Autodesk Inventor part; units mm, degrees
ref_plane "Work Plane1" through (26.5484, 0, 0) normal (0, 0, -1) x (-1, 0, 0)
ref_plane "YZ Plane" through (0, 0, 0) normal (1, 0, 0) x (0, 1, 0)
ref_plane "XZ Plane" through (0, 0, 0) normal (0, 1, 0) x (-1, 0, 0)
sketch "Sketch1" plane through (0, 0, 0) normal (0, 0, 1) x (1, 0, 0)
  line L0 (-1.8762, 0) -> (9.646, 0)
  line L1 (3.3073, 6.5) -> (2.2392, 8.35)
  line L2 (3.3073, 6.5) -> (8, 6.5) construction
  line L3 (8, 6.5) -> (8, 0) construction
  arc A0 (2.2392, 8.35) -> (0, 7.75) centre (1.2, 7.75) ccw
  line L4 (3.3073, 6.5) -> (3.3073, 0)
  line L5 (0, -1.8418) -> (0, 11.0509)
  point P0 (0, 0)
  dimension "d2" = 13
  dimension "d4" = 17.9
  dimension "d5" = 1.2
  dimension "d15" = 8
  dimension "d16" = 30
revolve "Ring" add sketch "Sketch1" angle 360 about axis through (-10, 0, 0) along (1, 0, 0)
sketch "Sketch2" plane through (0, 0, 0) normal (-1, 0, 0) x (0, 0, 1)
  circle A0 centre (0, 0) radius 4.9
  line L0 (-6.5, -3.7528) -> (-6.5, 3.7528)
  line L1 (-6.5, 3.7528) -> (0, 7.5056)
  line L2 (0, 7.5056) -> (6.5, 3.7528)
  line L3 (6.5, 3.7528) -> (6.5, -3.7528)
  line L4 (6.5, -3.7528) -> (0, -7.5056)
  line L5 (0, -7.5056) -> (-6.5, -3.7528)
  circle A1 centre (0, 0) radius 7.75
  dimension "d6" = 15.0111
extrude "Body" add sketch "Sketch2" against normal blind 8 contours A0 | L0 L1 L2 L3 L4 L5
sketch "Sketch3" plane through (0, 0, 0) normal (0, 0, 1) x (1, 0, 0)
  line L0 (2.7268, 7.5056) -> (8, 7.5056)
  line L1 (8, 3.7528) -> (8, 7.5056)
  line L2 (0, -7.75) -> (0, 7.75)
  line L3 (-1.6, 0) -> (9.6, 0)
  line L4 (7.4194, 7.5056) -> (8, 6.5)
  dimension "d10" = 30
  dimension "d11" = 13
revolve "Chamfer1" cut sketch "Sketch3" angle 360 about axis through (-10, 0, 0) along (1, 0, 0)
sketch "Sketch4" plane through (0, 0, 0) normal (-1, 0, 0) x (0, 0, 1)
  circle A0 centre (0, 0) radius 7.75
hole "Thread" at (0, 0, 0) direction (1, 0, 0) diameter 6.647 end through all
chamfer "Chamfer2" distance 0.6766 angle 30 1 edges at (0, 0, -3.3235) measured on face at (0, 6.1914, -0.7518)
ref_plane "Work Plane1" through (26.5484, 0, 0) normal (0, 0, -1) x (-1, 0, 0)
chamfer "Chamfer3" distance 0.6766 angle 45 1 edges at (8, 0, -3.3235)
equation "\"d2\" = SW"
equation "\"d4\" = LADI"
equation "\"d5\" = PHH"
equation "\"d15\" = KOH"
equation "\"d16\" = KEWI"
equation "\"d6\" = 1.1547 * SW"
equation "\"d7\" = KOH"
equation "\"d10\" = ANG1"
equation "\"d11\" = SW0"
equation "\"d12\" = -0.5 * GD1 + 0.5 * NND"
equation "\"d46\" = -0.5 * GD1 + 0.5 * NND"
equation "\"d51\" = -0.5 * GD1 + 0.5 * NND"
equation "\"ANG1\" = 30deg"
equation "\"KEWI\" = 30deg"
equation "\"NND\" = 8"
equation "\"LADI\" = 17.9"
equation "\"SW\" = 13"
equation "\"PHH\" = RR"
equation "\"KOH\" = 8"
equation "\"SW0\" = SW"
equation "\"d1\" = LADI"
equation "\"d3\" = PHH"
equation "\"GUL\" = 0.541266 * PTC"
equation "\"RR\" = 1.2"
equation "\"THREADDIA\" = 8"
equation "\"TOA\" = 30deg"
equation "\"PTC\" = 1.25"
equation "\"RR1\" = 0.5"
equation "\"GAL\" = 0.541266 * PTC"
equation "\"E0\" = 1.155 * SW"
properties part number "ANSI B18.2.4.4M - M8 x 1,25" material "Steel, Mild"
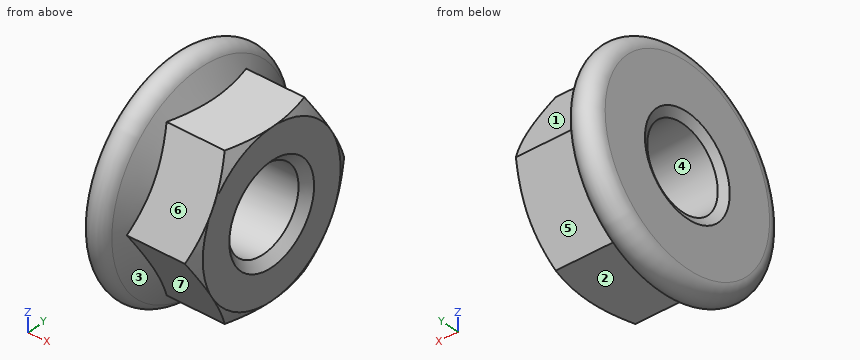
Verification items for the finished model (mm, model axes). Face numbers are marked on the shaded views. A direction names the side the tool comes from. Coordinates: 2 decimals unless noted, no trailing zeros. Loops run counter-clockwise (first coordinate to the right, second up) from the corner with the lowest first, then second, coordinate; pieces in that order, holes last. Notation, with made-up numbers: (42, 87.5) -> (56, 87.5) arc R33 ccw to (56, 122.5) -> close; hole circle Ø4 at (-30, -17.75). An arc over 180 degrees is marked (long way). Write each question's results on one line, items separated by ' | '.
Item 1: Mould release check, pull along Z, two halves, no side actions. Record for the marked faces 1, 2, 3 and 4: +Z half, -Z half, draft (parallel to the pull), parting line (faces both ways), or undercut.
Found:
face 1: +Z half | face 2: -Z half | face 3: parting line | face 4: undercut
Item 2: Section check B-B, the plane x = 1.5. Enter the section's corners in (y, z).
Found:
outline: circle Ø17.82 at (0, 0); hole circle Ø6.65 at (0, 0)
Item 3: Tool access check on the marked faces 5, 6 and 7. Record the directions out of +Z, -Z, +X, -X, +Y, -Y that give a thin tool (end or side, any length) a straight path to the whole face; none if there is none.
Found:
face 5: -Z, +X, +Y | face 6: +Z, +X, -Y | face 7: -Z, +X, -Y
Item 4: Gauge pin test, flat ends, axial feed: pin 1 (4 mm diameter, centred on y = -3, z = -1.5, fed in from +X); pin 2 (4 mm diameter, centred on x = 6, y = -1.5, fed in from -Z); pin 3 (2 mm diameter, centred on x = 7, z = 4.5, fed in from +Y); pin 4 (4 mm diameter, centred on x = 6.5, z = -5, fed in from -Y). Record the tip position at first contact, or that the pin passes through.
Found:
pin 1: stops at x = 8 | pin 2: stops at z = -6.5 | pin 3: stops at y = 5.48 | pin 4: stops at y = -5.77
Item 5: Material ranges on L1, parallel to Z at x = 4, y = 0; L2, parallel to Z at x = 1, y = -2.25; L3, parallel to Y at x = 6.5, z = -2.75, recorded low to high.
Found:
L1: z = -6.5 to -3.32, 3.32 to 6.5 | L2: z = -8.65 to -2.45, 2.45 to 8.65 | L3: y = -5.92 to -1.87, 1.87 to 5.92
Item 6: Section check A-A, the plane x = 5.5. Enter the section's corners in (y, z), plus the area to 3 significant figures.
Found:
outline: (-7.51, 0) -> (-3.75, -6.5) -> (3.75, -6.5) -> (7.51, 0) -> (3.75, 6.5) -> (-3.75, 6.5) -> close; hole circle Ø6.65 at (0, 0) | area: 112 mm2
